Autodesk Inventor part; units mm, degrees
ref_plane "YZ Plane" through (0, 0, 0) normal (1, 0, 0) x (0, 1, 0)
ref_plane "XZ Plane" through (0, 0, 0) normal (0, 1, 0) x (-1, 0, 0)
ref_plane "XY Plane" through (0, 0, 0) normal (0, 0, 1) x (1, 0, 0)
sketch "Sketch1" plane through (0, 0, 0) normal (0, 0, 1) x (1, 0, 0)
  circle A0 centre (0, 0) radius 8.75
  circle A1 centre (0, 0) radius 2.5
  dimension "d0" = 17.5
  dimension "d1" = 5
extrude "Extrusion1" add sketch "Sketch1" along normal blind 8
sketch "Sketch2" plane through (0, 0, 8) normal (0, 0, 1) x (1, 0, 0)
  circle A0 centre (0, 0) radius 2.5
  circle A1 centre (0, 0) radius 8.75
  circle A2 centre (0, 0) radius 10.5
  dimension "d4" = 21
extrude "Extrusion2" add sketch "Sketch2" along normal blind 1.6 contours A1 | A2
sketch "Sketch3" plane through (0, 0, 0) normal (0, 0, -1) x (-1, 0, 0)
  circle A0 centre (0, 0) radius 2.5
  circle A1 centre (0, 0) radius 8.75
  circle A2 centre (0, 0) radius 10.5
  dimension "d7" = 21
extrude "Extrusion3" add sketch "Sketch3" along normal blind 1.6 contours A1 | A2
sketch "Sketch5" plane through (0, 0, -1.6) normal (0, 0, -1) x (-1, 0, 0)
  circle A0 centre (0, 0) radius 2.5
  circle A1 centre (0, 0) radius 10.5
  circle A2 centre (0, 0) radius 8
  dimension "d11" = 16
extrude "Extrusion4" cut sketch "Sketch5" against normal blind 11 contours A2
properties part number "MSK01-06" material "Nylon-6/6"
Can you work these out from the model? Positions are in its coordinate system, mm. A direction names the side the tool comes from. Coordinates: 2 decimals unless noted, no trailing zeros. Order: outer loops, then holes, each group sorted by start corner. A loop starts at its lowest first (then second) coordinate and runs counter-clockwise, first axis right, second up.
1. Thinking about a two-plate mould opening in Z: for faces 4 (the face through (2, -8, -1.6)), 5 (the face through (2, -2, 9.6)), 6 (the face through (-4, 8, 8)), which applies, +Z half, -Z half, draft (parallel to the pull), parting line (faces both ways), or undercut?
2. For faces 1 (the face through (10, -3.2, 8.8)), 2 (the face through (-6.944, 5.324, 3.944)), 3 (the face through (1.73, -7.81, 3.82)), which set-ups out of +Z, -Z, +X, -X, +Y, -Y let a thin tool reach every point of the face, with its end or its side?
3. If we section it at D-D (x = -7): Please give me the cut outline in (y, z).
4. I'm going to push flat-ended pins straight in: pin 1 (1.5 mm diameter, centred on x = 5, y = -1.5, fed in from -Z); pin 2 (5 mm diameter, centred on y = -3, z = 2, fed in from +X); pin 3 (4 mm diameter, centred on x = 3.5, z = 0.5, fed in from -Y). Where does each tip first touch, or does it pass through?
5. If we section it at A-A (x = 0): Please give me the cut outline in (y, z), then the cut area to 3 significant figures.
6. I need wall thicknesses on line 1 (Z direction, x = -8.5, y = -6); line 2 (Y direction, x = 0, z = 9.5); line 3 (Y direction, x = 0, z = 6.5). Which ranges of each line are inside material? Lowest first, please.
7. If we section it at C-C (z = 8.75): Please give me the cut outline in (x, y), then the cut area to 3 significant figures.
Entries:
1. face 4: -Z half
1. face 5: +Z half
1. face 6: undercut
2. face 1: +Z, -Z
2. face 2: none
2. face 3: -Z
3. outline: (-7.83, -1.6) - (-3.87, -1.6) - (-3.87, 9.4) - (3.87, 9.4) - (3.87, -1.6) - (7.83, -1.6) - (7.83, 0) - (5.25, 0) - (5.25, 8) - (7.83, 8) - (7.83, 9.6) - (-7.83, 9.6) - (-7.83, 8) - (-5.25, 8) - (-5.25, 0) - (-7.83, 0) - close
4. pin 1: stops at z = 9.4
4. pin 2: stops at x = 10.39
4. pin 3: stops at y = -10.38
5. outline: (-10.5, -1.6) - (-8, -1.6) - (-8, 9.4) - (-2.5, 9.4) - (-2.5, 9.6) - (-10.5, 9.6) - (-10.5, 8) - (-8.75, 8) - (-8.75, 0) - (-10.5, 0) - close; (2.5, 9.4) - (8, 9.4) - (8, -1.6) - (10.5, -1.6) - (10.5, 0) - (8.75, 0) - (8.75, 8) - (10.5, 8) - (10.5, 9.6) - (2.5, 9.6) - close
5. area: 30.2 mm2
6. line 1: z = -1.6 to 0, 8 to 9.6
6. line 2: y = -10.5 to -2.5, 2.5 to 10.5
6. line 3: y = -8.75 to -8, 8 to 8.75
7. outline: circle Ø21 at (0, 0); hole circle Ø16 at (0, 0)
7. area: 145 mm2
